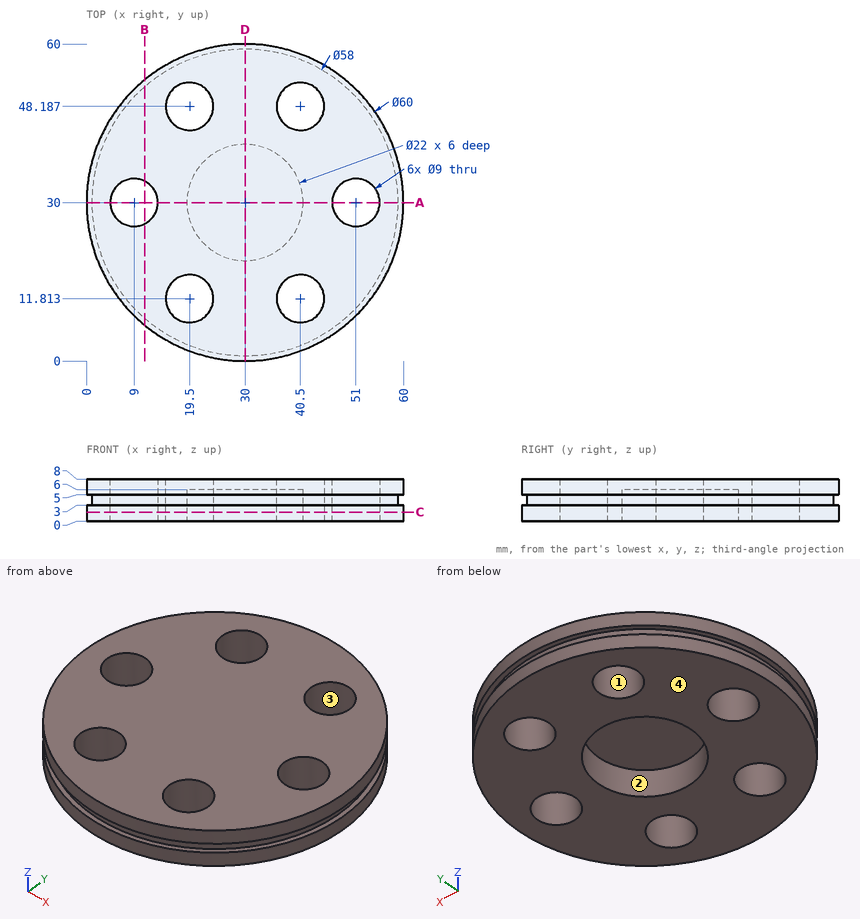
Input: dimensioned drawing with shaded views. Units: mm. Origin: part minimum x, y, z. A direction names the side the tool comes from. Round coordinates to 2 decimals unless told otherwise and drop trailing zeros. Loops run counter-clockwise (first coordinate to the right, second up) from the corner with the lowest first, then second, coordinate; pieces in that order, holes last. Notation, with made-up numbers: (-21.75, 15) -> (2.25, 15) arc R26 ccw to (2.25, 30) -> close; hole circle Ø11 at (2, 10.25). An arc over 180 degrees is marked (long way). Answer as a JSON object with one key per item and string values. Group by question number.
Q1. Access query for the marked faces 1 and 2. Directions: +Z, -Z, +X, -X, +Y, -Y. A direction counts if a zero-diameter tool reaches every point of the face in a straight line with its end or side. Return the directions, or none.
Q2. Section query A-A (y = 30). Output: boundary loops of the cut face in (x, z).
Q3. Section query D-D (x = 30). Output: boundary loops of the cut face in (y, z), plus the area to 3 significant figures.
Q4. Section query C-C (z = 1.75). Output: boundary loops of the cut face in (x, y), plus the area to 3 significant figures.
Q5. Contact query for flat-ended pins moving along their axis: P1, Ø5.5, axis at x = 19.5, y = 48.19, coming from the -Z side; P2, Ø11, axis at x = 28, y = 28.5, coming from the -Z side; P3, Ø1, axis at y = 20.5, z = 3, coming from the +X side. Output: stop coordinate, or through.
Q6. Mould query, pull axis Y, two halves, no side actions, for the marked faces 3 and 4. Classes: pulls with the +Y half, pulls with the -Y half, needs draft (parallel to the pull), parting line crosses it, or undercut.
Q7. Section query B-B (x = 11). Output: boundary loops of the cut face in (y, z), plus the area to 3 significant figures.
Q8. Ray query, line 1 (X direction, y = 11, z = 4.75) (1 decimal); line 2 (X direction, y = 47, z = 3.5) (1 decimal); line 3 (X direction, y = 29, z = 3.5) (1 decimal). Return the intervals inside material, ascending. Write a range as from..to.
Completed:
{
 "1": {"face 1": "+Z, -Z", "face 2": "-Z"},
 "2": {"outline": "(0, 0) -> (4.5, 0) -> (4.5, 8) -> (0, 8) -> (0, 5) -> (1, 5) -> (1, 3) -> (0, 3) -> close; (13.5, 0) -> (19, 0) -> (19, 6) -> (41, 6) -> (41, 0) -> (46.5, 0) -> (46.5, 8) -> (13.5, 8) -> close; (55.5, 0) -> (60, 0) -> (60, 3) -> (59, 3) -> (59, 5) -> (60, 5) -> (60, 8) -> (55.5, 8) -> close"},
 "3": {"outline": "(0, 0) -> (19, 0) -> (19, 6) -> (41, 6) -> (41, 0) -> (60, 0) -> (60, 3) -> (59, 3) -> (59, 5) -> (60, 5) -> (60, 8) -> (0, 8) -> (0, 5) -> (1, 5) -> (1, 3) -> (0, 3) -> close", "area": "344 mm²"},
 "4": {"outline": "circle Ø60 at (30, 30); hole circle Ø9 at (9, 30); hole circle Ø9 at (19.5, 11.81); hole circle Ø9 at (19.5, 48.19); hole circle Ø22 at (30, 30); hole circle Ø9 at (40.5, 11.81); hole circle Ø9 at (40.5, 48.19); hole circle Ø9 at (51, 30)", "area": "2,070 mm²"},
 "5": {"P1": "through", "P2": "z = 6", "P3": "x = 58.62"},
 "6": {"face 3": "undercut", "face 4": "needs draft"},
 "7": {"outline": "(6.78, 0) -> (25.97, 0) -> (25.97, 8) -> (6.78, 8) -> (6.78, 5) -> (8.09, 5) -> (8.09, 3) -> (6.78, 3) -> close; (34.03, 0) -> (53.22, 0) -> (53.22, 3) -> (51.91, 3) -> (51.91, 5) -> (53.22, 5) -> (53.22, 8) -> (34.03, 8) -> close", "area": "302 mm²"},
 "8": {"line 1": "8.1..15.1, 23.9..36.1, 44.9..51.9", "line 2": "6.5..15.2, 23.8..36.2, 44.8..53.5", "line 3": "1..4.6, 13.4..19, 41..46.6, 55.4..59"}
}
